from build123d import *

# Parameters (mm, degrees)
BOSS_EXTRUDE1_DEPTH      = 25
BOSS_EXTRUDE1_DEPTH_BACK = 2.5
SKETCH1_W                = 68
SKETCH1_H                = 88
SKETCH2_W                = 82.510400987
SKETCH2_H                = 84
CUT_EXTRUDE1_DEPTH       = 25
SKETCH3_W                = 23
SKETCH3_H                = 25
CUT_EXTRUDE2_DEPTH       = 25
SKETCH4_W                = 20
SKETCH4_H                = 25
CUT_EXTRUDE3_DEPTH       = 25
FILLET2_R                = 10


with BuildPart() as part:
    # Sketch1 → Boss-Extrude1 (new, two sides: drawn at the far end of the back side and taken through both)
    with BuildSketch(Plane.XY.offset(-BOSS_EXTRUDE1_DEPTH_BACK)):
        with Locations((-34, -44)):
            Rectangle(SKETCH1_W, SKETCH1_H)
    extrude(amount=BOSS_EXTRUDE1_DEPTH + BOSS_EXTRUDE1_DEPTH_BACK)

    # Sketch2 → Cut-Extrude1 (cut)
    with BuildSketch(Plane.XY.offset(25)):
        with Locations((-33.923509309, -44)):
            Rectangle(SKETCH2_W, SKETCH2_H)
    extrude(amount=-CUT_EXTRUDE1_DEPTH, mode=Mode.SUBTRACT)

    # Sketch3 → Cut-Extrude2 (cut)
    with BuildSketch(Plane(origin=(0, 0, 0), x_dir=(1, 0, 0), z_dir=(0, 1, 0))):
        with Locations((-56.5, -12.5)):
            Rectangle(SKETCH3_W, SKETCH3_H)
    extrude(amount=-CUT_EXTRUDE2_DEPTH, mode=Mode.SUBTRACT)

    # Sketch4 → Cut-Extrude3 (cut)
    with BuildSketch(Plane(origin=(0, 0, 0), x_dir=(1, 0, 0), z_dir=(0, 1, 0))):
        with Locations((-10, -12.5)):
            Rectangle(SKETCH4_W, SKETCH4_H)
    extrude(amount=-CUT_EXTRUDE3_DEPTH, mode=Mode.SUBTRACT)

    # Fillet2
    fillet2_edges = [part.edges().sort_by_distance(p)[0] for p in [
        (-34, -86, 0),
        (-32.5, -2, 0),
    ]]
    fillet(fillet2_edges, radius=FILLET2_R)


solid = part.part
Work out the finished part from the listing and answer in its coordinate system (mm). A direction names the side the tool comes from. Round coordinates to 2 decimals unless told otherwise and drop trailing zeros. Order: outer loops, then holes, each group sorted by start corner. A loop starts at its lowest first (then second) coordinate and runs counter-clockwise, first axis right, second up. Notation, with made-up numbers: M -31.75,-28 L 17.25,-28 A29 cw 17.25,4 Z; hole C -29.75,-19 d11. An arc over 180 degrees is marked long. Put each result on its own line as item: value. Start each with the question number.
Q1. Section A-A, the plane z = 12.5 is taken. Write down the section's boundary in (x, y), and give its area (3 significant figures).
Q2. Flat-ended cylindrical pins translate along their axes: pin 1 (5 mm diameter, centred on x = -60.5, y = -45, fed in from +Z); pin 2 (4 mm diameter, centred on y = -29, z = 2.5, fed in from +X); pin 3 (12 mm diameter, centred on x = -57.5, z = 18, fed in from +Y); pin 4 (10 mm diameter, centred on x = -61, z = 4, fed in from +Y). Find the tip coordinate at first contact, or state that the pin passes through.
Q3. Section C-C, the plane x = -18 is taken. Write down the section's boundary in (y, z), and give its area (3 significant figures).
Q4. A tool of negligible diameter and unlimited length cuts with its end or side. For faces 5 (the flat face through (0, -54, -1)), 6 (the flat face through (-45, -1.5, 10.7)), 7 (the flat face through (-20, -1.5, 10.7)), 8 (the cylindrical face through (-32.33, -4.85, 3.01)), from which of +Z, -Z, +X, -X, +Y, -Y can it reach the whole face along a straight path? Write none if from no direction.
Q5. Straight lines are drawn through the part: L1, parallel to Y at x = -23, z = 10.75; L2, parallel to Y at x = -14.5, z = 13; L3, parallel to Z at x = -57, y = -39. For each, find the intervals that lie inside material, in ascending order. Write a range as [from, to].
Q6. For a pull along Y with two mould halves and no side action, classify faces 1 (the flat face through (-34, -87, 25)), 2 (the flat face through (-34, 0, 8)), 3 (the flat face through (-34, -86, 18)), 4 (the flat face through (-33, -2, 18)) as pulls with the +Y half, pulls with the -Y half, needs draft (parallel to the pull), parting line crosses it, or undercut.
Q7. Section D-D, the plane y = -13 is taken. Write down the section's boundary in (x, z).
Q8. Section B-B, the plane z = 2 is taken. Write down the section's boundary in (x, y).
Findings below:
1. outline: M -68,-88 L 0,-88 L 0,-86 L -68,-86 Z; M -45,-2 L -20,-2 L -20,0 L -45,0 Z
1. area: 186 mm^2
2. pin 1: stops at z = 0
2. pin 2: passes through
2. pin 3: stops at y = -86
2. pin 4: stops at y = 0
3. outline: M -88,-2.5 L 0,-2.5 L 0,0 L -76,0 A10 cw -86,10 L -86,25 L -88,25 Z
3. area: 291 mm^2
4. face 5: +Z, -Z, +X, +Y, -Y
4. face 6: +Z, -X, +Y
4. face 7: +Z, +X, +Y
4. face 8: +Z, +X, -X
5. L1: y = [-88, -86], [-2, 0]
5. L2: y = [-88, -86]
5. L3: z = [-2.5, 0]
6. face 1: needs draft
6. face 2: pulls with the +Y half
6. face 3: undercut
6. face 4: undercut
7. outline: M -68,-2.5 L 0,-2.5 L 0,0 L -68,0 Z
8. outline: M -68,-88 L 0,-88 L 0,-82 L -68,-82 Z; M -45,-6 L -20,-6 L -20,0 L -45,0 Z
